from build123d import *

# Parameters (mm, degrees)
F0_W     = 75
F0_H     = 105
F0_W_2   = 5
F1_DEPTH = 10
F2_T     = -5
F4_DEPTH = 25
F5_DEPTH = 10
F6_W     = 2.5
F6_H     = 4
F7_DEPTH = 25


with BuildPart() as f1:
    # F0 (on Top) → F1 (new body)
    with BuildSketch(Plane.XY):
        with Locations((40, 0)):
            Rectangle(F0_W, F0_H)
        with Locations((-40, 0)):
            Rectangle(F0_W, F0_H)
        Rectangle(F0_W_2, F0_H)
    extrude(amount=F1_DEPTH)

    # F2
    f2_openings = [f1.faces().sort_by_distance(p)[0] for p in [
        (0, 0, 10),
    ]]
    offset(amount=F2_T, openings=f2_openings)

    # F3 (on Top) → F4 (intersect)
    with BuildSketch(Plane.XY):
        Polygon((-67.5, 52.5), (-77.5, 52.5), (-77.5, -52.5), (-67.5, -52.5), (-67.5, -47.5), (-62.5, -47.5), (-62.5, -52.5), (62.5, -52.5), (62.5, -47.5), (67.5, -47.5), (67.5, -52.5), (77.5, -52.5), (77.5, 52.5), (67.5, 52.5), (67.5, 47.5), (62.5, 47.5), (62.5, 52.5), (-62.5, 52.5), (-62.5, 47.5), (-67.5, 47.5), align=None)
    extrude(amount=F4_DEPTH, mode=Mode.INTERSECT)

    # F0 (on Top) → F5 (join)
    with BuildSketch(Plane.XY):
        Rectangle(F0_W_2, F0_H)
    extrude(amount=F5_DEPTH)

    # F6 (on face) → F7 (cut)
    with BuildSketch(Plane(origin=(-2.5, 0, 0), x_dir=(0, -1, 0), z_dir=(-1, 0, 0))):
        with Locations((-1.25, 7)):
            Rectangle(F6_W, F6_H)
        with Locations((1.25, 7)):
            Rectangle(F6_W, F6_H)
    extrude(amount=-F7_DEPTH, mode=Mode.SUBTRACT)


solid = f1.part
The model under review builds one solid part; all positions refer to its coordinate system, in mm. A direction names the side the tool comes from. Give positions to 0.01 mm unless a question says otherwise; leave off trailing zeros. Write each loop counter-clockwise with the first axis right and the second up, starting at its lowest first coordinate (ties: lowest second). Pieces come first, ordered by that corner, then holes. Notation, with made-up numbers: M -5.5,-33 L 25.5,-33 A20 cw 25.5,-27 Z; hole C 36.25,0 d11. An arc over 180 degrees is marked long. One line per question, with ' | ' between items. Start each with the question number.
Item 1: Draft analysis for pull direction Y (two halves, no side actions). For faces 4 (the flat face through (72.5, -1, 7)), 5 (the flat face through (65, 47.5, 2)), 6 (the flat face through (70, -47.5, 7)), 7 (the flat face through (-62.5, 50, 5)), state which applies: released by +Y, released by -Y, zero draft, split by the parting line, or undercut.
Item 2: We need section B-B on y = -10.5. Write out the cut boundary in (x, z), plus the area to 3 significant figures.
Item 3: We need section A-A on x = -0.5. Write out the cut boundary in (y, z).
Item 4: Wall thickness on line 1 (X direction, y = 13, z = 6.5); line 2 (Y direction, x = -36.5, z = 6.25); line 3 (X direction, y = -1, z = 8.5): over which ranges is each line inside the solid? List them lowest first. Write a range as from..to.
Item 5: For faces 1 (the flat face through (62.5, -50, 5)), 2 (the flat face through (0, 0, 10)), 3 (the flat face through (-32, 47.5, 7)), list the 3-axis set-ups (+Z, -Z, +X, -X, +Y, -Y) from which the entire face can be reached by the end or side of a thin tool; tool diameter is ignored.
Item 6: For pin 1 (2 mm diameter, centred on x = -14, y = 13.5, fed in from +Z); pin 2 (2.5 mm diameter, centred on x = -64.5, z = 3, fed in from -Y), all flat-tipped, find the tip position at first contact; note any pin that passes through.
Results found:
1) face 4: undercut | face 5: released by +Y | face 6: undercut | face 7: zero draft
2) outline: M -77.5,0 L 77.5,0 L 77.5,10 L 72.5,10 L 72.5,5 L 2.5,5 L 2.5,10 L -2.5,10 L -2.5,5 L -72.5,5 L -72.5,10 L -77.5,10 Z | area: 850 mm2
3) outline: M -52.5,0 L 52.5,0 L 52.5,10 L -52.5,10 Z; hole M -2.5,5 L 2.5,5 L 2.5,9 L -2.5,9 Z
4) line 1: x = -77.5..-72.5, -2.5..2.5, 72.5..77.5 | line 2: y = -52.5..-47.5, 47.5..52.5 | line 3: x = -77.5..-72.5, 72.5..77.5
5) face 1: +Z, -Z, -Y | face 2: +Z, +X, -X, +Y, -Y | face 3: +Z
6) pin 1: stops at z = 5 | pin 2: stops at y = -47.5
